Design review of the part built by this model. Coordinates are the model's own, in mm. A direction names the side the tool comes from. Round coordinates to 2 decimals unless told otherwise and drop trailing zeros. Write each loop counter-clockwise with the first axis right and the second up, starting at its lowest first coordinate (ties: lowest second). Pieces come first, ordered by that corner, then holes. Notation, with made-up numbers: (66.25, -2.75) -> (84.25, -2.75) arc R36 cw to (84.25, 32.25) -> close; hole circle Ø3 at (-28.5, 14.25). An arc over 180 degrees is marked (long way). One line per question, with ' | ' between items. Start each with the question number.
1) Mouldability with a two-part tool opening along X and no side actions: class faces 1 (the flat face through (29, 32, 0)), 2 (the flat face through (-18, 2, 16)), 3 (the flat face through (29, 67, 8)) as +X half, -X half, draft (parallel to the pull), parting line (faces both ways), or undercut.
2) Insertion check: pin 1 Ø8 at (x, y) = (27.5, 57.5) entering from +Z; pin 2 Ø5 at (x, y) = (-12.5, 60) entering from -Z; pin 3 Ø5 at (y, z) = (19, 2.5) entering from -X; pin 4 Ø6 at (x, z) = (-3.5, 8) entering from -Y. Each pin has a flat end and moves straight along its axis. Give the tip position at first contact, or say it passes through.
3) Consider section C-C (y = 17). Give the boundary of the cut face in (x, z).
4) Consider section B-B (x = -8). Give the boundary of the cut face in (y, z), then the cut area to 3 significant figures.
5) For probe 1 along Y at (x, z) = (-8, 16.8); probe 2 along Y at (x, z) = (22.5, 16.5); probe 3 along X at (y, z) = (63, 0.25), list the stretches that pass through material, from the lowest coordinate up.
6) Consider section D-D (z = 4). Give the boundary of the cut face in (x, y), then the cut area to 3 significant figures.
7) For faces 4 (the flat face through (0, 32, 9)), 5 (the flat face through (-10, 62, 14)), 6 (the cylindrical face through (61, 19, 4)), 7 (the flat face through (69, 57, 17)), 8 (the flat face through (69, 2, 14)), list the 3-axis set-ups (+Z, -Z, +X, -X, +Y, -Y) from which the entire face can be reached by the end or side of a thin tool; tool diameter is ignored.
8) Consider section A-A (y = 62). Give the boundary of the cut face in (x, z).
```python
from build123d import *

# Parameters (mm, degrees)
SKETCH1_W           = 59
SKETCH1_H           = 64
BOSS_EXTRUDE1_DEPTH = 19
SHELL1_T            = 3
SKETCH2_R           = 2
CUT_EXTRUDE1_DEPTH  = 19
SKETCH3_W           = 5
SKETCH3_H           = 10
BOSS_EXTRUDE2_DEPTH = 15
SKETCH4_W           = 5
SKETCH4_H           = 10
BOSS_EXTRUDE3_DEPTH = 15
SKETCH5_R           = 1.5
CUT_EXTRUDE2_DEPTH  = 10


with BuildPart() as part:
    # Sketch1 → Boss-Extrude1 (new body)
    with BuildSketch(Plane.XY):
        with Locations((29.5, 32)):
            Rectangle(SKETCH1_W, SKETCH1_H)
    extrude(amount=BOSS_EXTRUDE1_DEPTH)

    # Shell1
    shell1_openings = [part.faces().sort_by_distance(p)[0] for p in [
        (29.5, 32, 19),
    ]]
    offset(amount=SHELL1_T, openings=shell1_openings, kind=Kind.INTERSECTION)

    # Sketch2 → Cut-Extrude1 (cut)
    with BuildSketch(Plane(origin=(62, 0, 0), x_dir=(0, 0, -1), z_dir=(1, 0, 0))):
        with Locations((-4, 17)):
            Circle(SKETCH2_R)
    extrude(amount=-CUT_EXTRUDE1_DEPTH, mode=Mode.SUBTRACT)

    # Sketch3 → Boss-Extrude2 (add)
    with BuildSketch(Plane(origin=(62, 0, 0), x_dir=(0, 0, -1), z_dir=(1, 0, 0))):
        with Locations((-16.5, 62)):
            Rectangle(SKETCH3_W, SKETCH3_H)
        with Locations((-16.5, 2)):
            Rectangle(SKETCH3_W, SKETCH3_H)
    extrude(amount=BOSS_EXTRUDE2_DEPTH)

    # Sketch4 → Boss-Extrude3 (add)
    with BuildSketch(Plane.ZY.offset(3)):
        with Locations((16.5, 2)):
            Rectangle(SKETCH4_W, SKETCH4_H)
        with Locations((16.5, 62)):
            Rectangle(SKETCH4_W, SKETCH4_H)
    extrude(amount=BOSS_EXTRUDE3_DEPTH)

    # Sketch5 → Cut-Extrude2 (cut)
    with BuildSketch(Plane(origin=(0, 0, 14), x_dir=(-1, 0, 0), z_dir=(0, 0, -1))):
        with Locations((-67, 62)):
            Circle(SKETCH5_R)
        with Locations((8, 2)):
            Circle(SKETCH5_R)
        with Locations((-67, 2)):
            Circle(SKETCH5_R)
        with Locations((8, 62)):
            Circle(SKETCH5_R)
    extrude(amount=-CUT_EXTRUDE2_DEPTH, mode=Mode.SUBTRACT)


solid = part.part
```
From the geometry:
1) face 1: undercut | face 2: -X half | face 3: draft
2) pin 1: stops at z = 0 | pin 2: stops at z = 14 | pin 3: stops at x = -3 | pin 4: stops at y = -3
3) outline: (-3, -3) -> (62, -3) -> (62, 2) -> (59, 2) -> (59, 0) -> (0, 0) -> (0, 19) -> (-3, 19) -> close; (59, 6) -> (62, 6) -> (62, 19) -> (59, 19) -> close
4) outline: (-3, 14) -> (0.5, 14) -> (0.5, 19) -> (-3, 19) -> close; (3.5, 14) -> (7, 14) -> (7, 19) -> (3.5, 19) -> close; (57, 14) -> (60.5, 14) -> (60.5, 19) -> (57, 19) -> close; (63.5, 14) -> (67, 14) -> (67, 19) -> (63.5, 19) -> close | area: 70.0 mm2
5) probe 1: y = -3 to 0.5, 3.5 to 7, 57 to 60.5, 63.5 to 67 | probe 2: y = -3 to 0, 64 to 67 | probe 3: x = -3 to 0, 59 to 62
6) outline: (-3, -3) -> (62, -3) -> (62, 15) -> (59, 15) -> (59, 0) -> (0, 0) -> (0, 64) -> (59, 64) -> (59, 19) -> (62, 19) -> (62, 67) -> (-3, 67) -> close | area: 762 mm2
7) face 4: +Z | face 5: -Z, -X, +Y, -Y | face 6: +X | face 7: +Z, -Z, +X | face 8: -Z, +X, +Y, -Y
8) outline: (-18, 14) -> (-9.5, 14) -> (-9.5, 19) -> (-18, 19) -> close; (-6.5, 14) -> (-3, 14) -> (-3, -3) -> (62, -3) -> (62, 14) -> (65.5, 14) -> (65.5, 19) -> (59, 19) -> (59, 0) -> (0, 0) -> (0, 19) -> (-6.5, 19) -> close; (68.5, 14) -> (77, 14) -> (77, 19) -> (68.5, 19) -> close
